```python
from build123d import *

# Parameters (mm, degrees)
F0_R     = 6.35
F1_DEPTH = 500
F3_DEPTH = 10
F5_DEPTH = 12.7


with BuildPart() as f1:
    # F0 (on Top) → F1 (new body)
    with BuildSketch(Plane.XY):
        Circle(F0_R)
    extrude(amount=F1_DEPTH)

    # F2 (on face) → F3 (join)
    with BuildSketch(Plane.XY.offset(500)):
        with BuildLine():
            Line((-4.0875947315, 4.8594309657), (-15.054643582, 17.89732251))
            Line((-15.054643582, 17.89732251), (-16.0928926438, 19.1316179753))
            ThreePointArc((-16.0928926438, 19.1316179753), (-25.5738890172, 18.1328072988), (-23.379079454, 8.855430192))
            Line((-23.379079454, 8.855430192), (-21.8707547639, 8.2841132578))
            Line((-21.8707547639, 8.2841132578), (-5.9382861813, 2.2492792688))
            ThreePointArc((-5.9382861813, 2.2492792688), (-5.1800381263, 3.6728333763), (-4.0875947315, 4.8594309657))
        make_face()
        with BuildLine():
            Line((18.109629911, 14.7985725966), (4.9170760776, 4.0180670536))
            ThreePointArc((4.9170760776, 4.0180670536), (5.7735991749, 2.6434924943), (6.2545341231, 1.096951641))
            Line((6.2545341231, 1.096951641), (23.8165818414, 4.1770718682))
            ThreePointArc((23.8165818414, 4.1770718682), (28.6497325197, 12.7023738091), (19.3585672347, 15.8191616282))
            Line((19.3585672347, 15.8191616282), (18.109629911, 14.7985725966))
        make_face()
        with BuildLine():
            Line((3.9393819064, -23.8570486481), (1.0345312657, -6.2651612158))
            ThreePointArc((1.0345312657, -6.2651612158), (-0.5907479446, -6.3224612981), (-2.1772790737, -5.96506126))
            Line((-2.1772790737, -5.96506126), (-8.2908405694, -22.7143008401))
            ThreePointArc((-8.2908405694, -22.7143008401), (-2.9165272541, -31.2140412119), (3.9393819064, -23.8570486481))
        make_face()
    extrude(amount=-F3_DEPTH)

    # F4 (on face) → F5 (cut)
    with BuildSketch(Plane(origin=(0, 0, 0), x_dir=(1, 0, 0), z_dir=(0, 0, -1))):
        with BuildLine():
            Line((1.27, -3.81), (0, -3.81))
            Line((0, -3.81), (0, -6.35))
            ThreePointArc((0, -6.35), (0.6382319087, -6.3178445716), (1.27, -6.2217039467))
            Line((1.27, -6.2217039467), (1.27, -3.81))
        make_face()
        with BuildLine():
            Line((0, -6.35), (0, -3.81))
            Line((0, -3.81), (-1.27, -3.81))
            Line((-1.27, -3.81), (-1.27, -6.2217039467))
            ThreePointArc((-1.27, -6.2217039467), (-0.6382319087, -6.3178445716), (0, -6.35))
        make_face()
    extrude(amount=-F5_DEPTH, mode=Mode.SUBTRACT)


solid = f1.part
```
The listing builds one solid part. Answer for the finished solid, in the listing's coordinates (mm). A direction names the side the tool comes from. Coordinates: 2 decimals unless noted, no trailing zeros. Write each loop counter-clockwise with the first axis right and the second up, starting at its lowest first coordinate (ties: lowest second). Pieces come first, ordered by that corner, then holes. Notation, with made-up numbers: M 73.5,3.5 L 98.5,3.5 A31 ccw 98.5,35.5 Z; hole C 57,30.25 d1. An arc over 180 degrees is marked long. Use a Markdown table: item, result. Add a question column.
1. Section B-B (y = -12) is taken. Give the vertices of the cut face in (x, z), plus the area to 3 significant figures.
2. Straight lines are drawn through the part: line 1 along Z through (x, y) = (-5, -28); line 2 along X through (y, z) = (-1, 442); line 3 along Y through (x, z) = (5, 446.5). For each, find the intervals that lie inside material, in ascending order. Write a range as [from, to].
3. Given P1, Ø0.8, axis at x = 0, y = 5, coming from the -Z side; P2, Ø1.9, axis at y = 4.5, z = 8, coming from the +X side (3 decimals); P3, Ø1, axis at y = 0, z = 249.5, coming from the -X side; P4, Ø2, axis at x = -4, y = 9, coming from the +Z side, each flat-ended and moving along its own axis, determine where each tip first touches the part or whether it passes through.
4. Which of the six approach directions +Z, -Z, +X, -X, +Y, -Y give full straight-line access (tool end or side, diameter ignored) to faces 1 (the cylindrical face through (-1.38, -6.2, 246.5)), 2 (the flat face through (2.507, -15.184, 495.07)), 3 (the flat face through (14.913, 2.615, 495.07)), 4 (the flat face through (-5.19, -14.22, 495.07))?
5. Section A-A (z = 350) is taken. Give the vertices of the cut face in (x, y).
Data:
| question | item | result |
|---|---|---|
| 1 | outline | M -4.38,490 L 1.98,490 L 1.98,500 L -4.38,500 Z |
| 1 | area | 63.6 mm2 |
| 2 | line 1 | z = [490, 500] |
| 2 | line 2 | x = [-6.27, 6.27] |
| 2 | line 3 | y = [-3.91, 3.91] |
| 3 | P1 | stops at z = 12.7 |
| 3 | P2 | stops at x = 5.265 |
| 3 | P3 | stops at x = -6.35 |
| 3 | P4 | passes through |
| 4 | face 1 | -Z |
| 4 | face 2 | +Z, -Z, +X |
| 4 | face 3 | +Z, -Z, +X, -Y |
| 4 | face 4 | +Z, -Z, -X |
| 5 | outline | C 0,0 d12.7 |
